Here's the drawing with two shaded views (mm, measured from the low corner). I have some questions. A direction names the side the tool comes from. Round coordinates to 2 decimals unless told otherwise and drop trailing zeros. Order: outer loops, then holes, each group sorted by start corner. A loop starts at its lowest first (then second) coordinate and runs counter-clockwise, first axis right, second up. Notation, with made-up numbers: (28, 78.5) -> (85, 78.5) arc R14 cw to (85, 103.5) -> close; hole circle Ø6 at (50, 12). An arc over 180 degrees is marked (long way). Put each result on its own line as item: value. Start each with the question number.
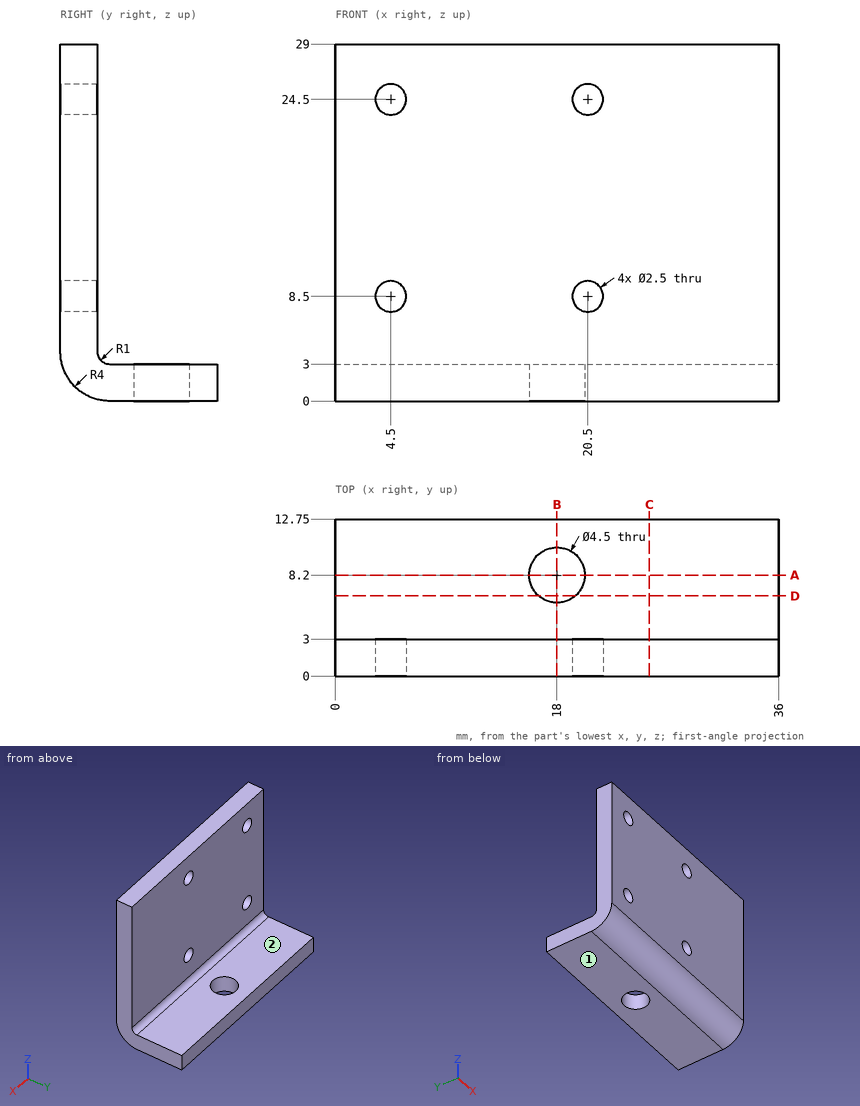
1. If we section it at D-D, the plane y = 6.5: Please give me the cut outline in (x, z).
2. If we section it at C-C, the plane x = 25.5: Please give me the cut outline in (y, z).
3. For pin 1 Ø4 at (x, y) = (13.5, 2) entering from -Z; pin 2 Ø2 at (x, z) = (20.5, 24.5) entering from -Y; pin 3 Ø8 at (x, z) = (27, 12.5) entering from +Y; pin 4 Ø2.5 at (x, y) = (23, 6.5) entering from +Z, each with a flat end and sliding along its axis, tell me the tip position at first contact or that it passes through.
4. Which directions (+Z, -Z, +X, -X, +Y, -Y) give clear straight access to the entire face, cutting with the end or side of a thin tool? Please do the marked faces 1 and 2.
5. If we section it at B-B, the plane x = 18: Please give me the cut outline in (y, z).
6. If we section it at A-A, the plane y = 8.2: Please give me the cut outline in (x, z).
7. I need wall thicknesses on L1, parallel to X at y = 1.65, z = 24.5; L2, parallel to Z at x = 4.5, y = 1.9; L3, parallel to Z at x = 7, y = 5. Which ranges of each line are inside material? Lowest first, please.
Results below:
1. outline: (0, 0) -> (16.53, 0) -> (16.53, 3) -> (0, 3) -> close; (19.47, 0) -> (36, 0) -> (36, 3) -> (19.47, 3) -> close
2. outline: (0, 4) arc R4 ccw to (4, 0) -> (12.75, 0) -> (12.75, 3) -> (4, 3) arc R1 cw to (3, 4) -> (3, 29) -> (0, 29) -> close
3. pin 1: z = 0
3. pin 2: through
3. pin 3: y = 3
3. pin 4: z = 3
4. face 1: -Z, +X, -X, +Y, -Y
4. face 2: +Z, +X, -X, +Y
5. outline: (0, 4) arc R4 ccw to (4, 0) -> (5.95, 0) -> (5.95, 3) -> (4, 3) arc R1 cw to (3, 4) -> (3, 29) -> (0, 29) -> close; (10.45, 0) -> (12.75, 0) -> (12.75, 3) -> (10.45, 3) -> close
6. outline: (0, 0) -> (15.75, 0) -> (15.75, 3) -> (0, 3) -> close; (20.25, 0) -> (36, 0) -> (36, 3) -> (20.25, 3) -> close
7. L1: 0 to 3.25, 5.75 to 19.25, 21.75 to 36
7. L2: 0.6 to 7.25, 9.75 to 23.25, 25.75 to 29
7. L3: 0 to 3
